Job drawing, mm, ordinate dimensions from the low corner. One solid piece. Coordinates: 2 decimals unless noted, no trailing zeros. Write each loop counter-clockwise with the first axis right and the second up, starting at its lowest first coordinate (ties: lowest second). Pieces come first, ordered by that corner, then holes. Notation, with made-up numbers: (71, 83) - (127, 83) arc R19 cw to (127, 119) - close; hole circle Ø11 at (26.5, 45.5). An arc over 180 degrees is marked (long way). Put each result on its own line as item: value. Start each with the question number.
1. Pull direction Y, two halves, no side cores. Call the marked faces 1, 2 and 3: released by +Y, released by -Y, zero draft, split by the parting line, or undercut.
2. Saw through at C-C, the plane x = 51.5. Write the cut outline in (y, z), plus the area to 3 significant figures.
3. Drop a flat-ended pin along its axis: P1, Ø1, axis at x = 8, z = 9, coming from the -Y side. Give the stop position or say it passes through.
4. Saw through at A-A, the plane z = 1. Write the cut outline in (x, y).
5. Saw through at D-D, the plane x = 16.25. Write the cut outline in (y, z), plus the area to 3 significant figures.
6. Drill centre lines: L1, parallel to X at y = 19.5, z = 6.5; L2, parallel to X at y = 16, z = 3.25; L3, parallel to Y at x = 43.75, z = 4.25. Where is each one in solid material? Low to high. Write a range as from..to.
7. Saw through at B-B, the plane y = 15. Write the cut outline in (x, z).
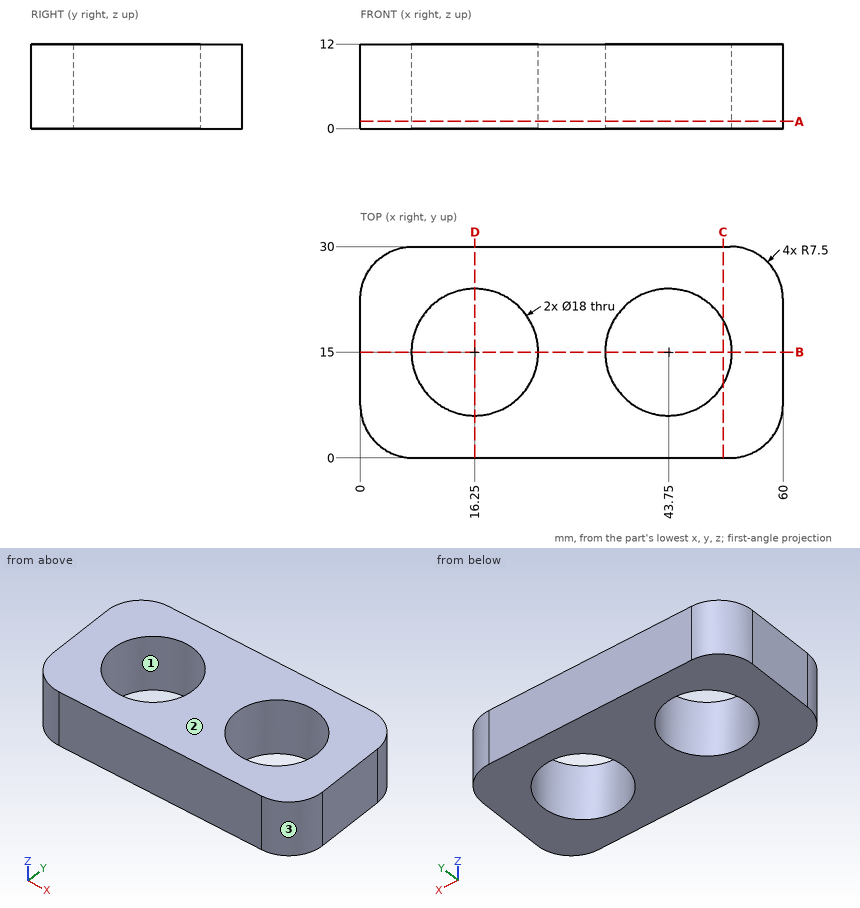
Final values:
1. face 1: undercut
1. face 2: zero draft
1. face 3: released by -Y
2. outline: (0, 0) - (10.42, 0) - (10.42, 12) - (0, 12) - close; (19.58, 0) - (30, 0) - (30, 12) - (19.58, 12) - close
2. area: 250 mm²
3. P1: stops at y = 0
4. outline: (0, 7.5) arc R7.5 ccw to (7.5, 0) - (52.5, 0) arc R7.5 ccw to (60, 7.5) - (60, 22.5) arc R7.5 ccw to (52.5, 30) - (7.5, 30) arc R7.5 ccw to (0, 22.5) - close; hole circle Ø18 at (16.25, 15); hole circle Ø18 at (43.75, 15)
5. outline: (0, 0) - (6, 0) - (6, 12) - (0, 12) - close; (24, 0) - (30, 0) - (30, 12) - (24, 12) - close
5. area: 144 mm²
6. L1: x = 0..8.46, 24.04..35.96, 51.54..60
6. L2: x = 0..7.31, 25.19..34.81, 52.69..60
6. L3: y = 0..6, 24..30
7. outline: (0, 0) - (7.25, 0) - (7.25, 12) - (0, 12) - close; (25.25, 0) - (34.75, 0) - (34.75, 12) - (25.25, 12) - close; (52.75, 0) - (60, 0) - (60, 12) - (52.75, 12) - close
